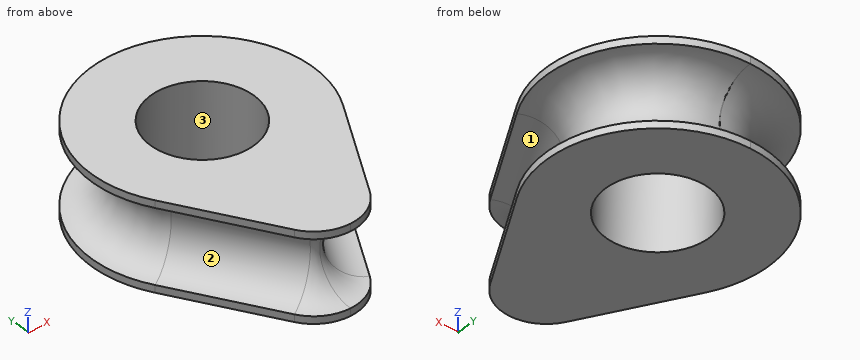
from build123d import *
from build123d import SkipClean  # not in build123d's __all__

# Parameters (mm, degrees)
F1_DEPTH = 6
F9_DEPTH = 25


with BuildPart() as f1:
    # F0 (on Top) → F1 (new body)
    with BuildSketch(Plane.XY):
        with BuildLine():
            Line((0, 3.5), (0, 7.5))
            ThreePointArc((0, 7.5), (-6.5081460588, 3.7274703054), (-6.4690456472, -3.7949240327))
            Line((-6.4690456472, -3.7949240327), (-2.5980762114, -10.4996397702))
            ThreePointArc((-2.5980762114, -10.4996397702), (-1.5, -11.5977159815), (0, -11.9996397702))
            Line((0, -11.9996397702), (0, -3.5))
            ThreePointArc((0, -3.5), (-3.5, 0), (0, 3.5))
        make_face()
    extrude(amount=F1_DEPTH)

    # F4: sweep along a path in F4_path
    with BuildLine(Plane(origin=(-2.5980762114, -10.4996397702, 0), x_dir=(0.5, -0.8660254038, 0), z_dir=(0.8660254038, 0.5, 0))) as f4_path:
        Line((0, 0), (-7.7419388717, 0))
    # F3 (on face) → F4 (sweep, cut)
    with BuildSketch(Plane(origin=(3.8969583329, -6.7497298276, 0), x_dir=(0.8660254038, 0.5, 0), z_dir=(0.5, -0.8660254038, 0))):
        with BuildLine():
            ThreePointArc((-7.4998198851, 0.5), (-4.9998198851, 3), (-7.4998198851, 5.5))
            Line((-7.4998198851, 5.5), (-7.4998198851, 0.5))
        make_face()
    sweep(path=f4_path.line, mode=Mode.SUBTRACT)

    # F7: sweep along a path in F0
    with BuildLine(Plane.XY) as f7_path:
        ThreePointArc((0, 7.5), (-6.5081460588, 3.7274703054), (-6.4690456472, -3.7949240327))
    # F6 (on face) → F7 (sweep, cut)
    with BuildSketch(Plane(origin=(0.0259888971, -0.0450140902, 0), x_dir=(-0.8660254038, -0.5, 0), z_dir=(-0.5, 0.8660254038, 0))):
        with BuildLine():
            ThreePointArc((7.4998198851, 5.5), (4.9998198851, 3), (7.4998198851, 0.5))
            Line((7.4998198851, 0.5), (7.4998198851, 5.5))
        make_face()
    sweep(path=f7_path.line, mode=Mode.SUBTRACT)

    # F8 (on face) → F9 (cut)
    with BuildSketch(Plane.YZ):
        with BuildLine():
            Line((7.5, 0.5), (7.5, 5.5))
            add(Edge.make_bspline(
                [(7.5, 5.5), (5.0000600383, 5.5), (5.0000600383, 3), (5.0000600383, 0.5), (7.5, 0.5)],
                knots=[0, 0, 0, 1.5707963268, 1.5707963268, 3.1415926536, 3.1415926536, 3.1415926536], degree=2, weights=[1, 0.7071067812, 1, 0.7071067812, 1]))
        make_face()
    extrude(amount=-F9_DEPTH, mode=Mode.SUBTRACT)

    # F11: sweep along a path in F0
    with BuildLine(Plane.XY) as f11_path:
        ThreePointArc((-2.5980762114, -10.4996397702), (-1.5, -11.5977159815), (0, -11.9996397702))
    # F10 (on face) → F11 (sweep, cut)
    with BuildSketch(Plane(origin=(3.8969583329, -6.7497298276, 0), x_dir=(-0.8660254038, -0.5, 0), z_dir=(-0.5, 0.8660254038, 0))):
        with BuildLine():
            ThreePointArc((7.4998198851, 5.5), (4.9998198851, 3), (7.4998198851, 0.5))
            Line((7.4998198851, 0.5), (7.4998198851, 5.5))
        make_face()
    sweep(path=f11_path.line, mode=Mode.SUBTRACT)

    # F12: F1 across plane


with BuildPart() as f1_1:
    add(f1.part, clean=False)
    with SkipClean():  # cleaning this boolean's faces spoils the solid; the shape is the same uncleaned
        add(f1.part.mirror(Plane.YZ), clean=False)


solid = f1_1.part
Model file for the job. Use its own axes, mm. Face numbers are marked on the shaded views. Coordinates: 2 decimals unless noted, no trailing zeros. Return JSON: item names as keys, results as strings.
1. Flat gauge pins, fed straight in: pin 1 (5 mm diameter, centred on x = 4, y = 0, fed in from -Z); pin 2 (2 mm diameter, centred on x = -3, z = 2.5, fed in from -Y). Where does each tip first touch, or does it go through?
Ans:
{"pin 1": "z = 0", "pin 2": "y = -6.73"}
2. Pull direction X, two halves, no side cores. Call the marked faces 1, 2 and 3: +X half, -X half, draft (parallel to the pull), parting line (faces both ways), or undercut.
Ans:
{"face 1": "+X half", "face 2": "-X half", "face 3": "undercut"}
3. Drill centre lines: probe 1 along X at (y, z) = (0, 2.3); probe 2 along X at (y, z) = (0.25, 2.9); probe 3 along Y at (x, z) = (-2.75, 1.45). Where is each one in solid material? Low to high.
Ans:
{"probe 1": "-5.1 to -3.5, 3.5 to 5.1", "probe 2": "-5 to -3.49, 3.49 to 5", "probe 3": "-6.31 to -2.17, 2.17 to 4.81"}
